Can you work these out from the model? Positions are in its coordinate system, mm. A direction names the side the tool comes from. Round coordinates to 2 decimals unless told otherwise and drop trailing zeros. Write each loop counter-clockwise with the first axis right and the second up, starting at its lowest first coordinate (ties: lowest second). Pieces come first, ordered by that corner, then holes.
Q1. We'd pull the mould along Y, two halves only. Please class faces 1 (the cylindrical face through (-29.414, 9.625, 35.14)), 2 (the flat face through (19, 99, 105)), 3 (the flat face through (5, 200, 42)), 4 (the flat face through (5, 0, 42)): +Y half, -Y half, draft (parallel to the pull), parting line (faces both ways), or undercut.
Q2. If we section it at C-C (z = 49): Please give me the cut outline in (x, y), plus the area to 3 significant figures.
Q3. If we section it at A-A (x = -26): Give the number of separate pieces and of enclosed holes in the cut face, plus the area to 3 significant figures.
Q4. If we section it at B-B (y = 53): Please give me the cut outline in (x, z), plus the area to 4 significant figures.
Q5. For faces 5 (the flat face through (-4, 99, 0)), 6 (the flat face through (0, 99, 75)), 7 (the cylindrical face through (-29.414, 59.625, 35.14)), which set-ups out of +Z, -Z, +X, -X, +Y, -Y let a thin tool reach every point of the face, with its end or its side?
Q6. I'm going to push flat-ended pins straight in: pin 1 Ø9.5 at (x, y) = (24, 75) entering from +Z; pin 2 Ø25 at (x, y) = (-24.5, 126) entering from +Z; pin 3 Ø23 at (x, y) = (-18.5, 140) entering from +Z. Where does each tip first touch, or does it pass through?
Q7. Please list where these lines run through material, in increasing order: line 1 along Y through (x, z) = (24, 94.25); line 2 along Y through (x, z) = (-26, 6.5); line 3 along X through (y, z) = (126, 36).
from build123d import *

# Parameters (mm, degrees)
F0_W           = 39
F0_H           = 60
F1_DEPTH       = 200
F4_D           = 15.5
F4_DEPTH       = 18
F4_TIP         = 4.6566697975
F5_D           = 22
F5_CBORE_D     = 31.5
F5_CBORE_DEPTH = 20


# Not quite as in the source:
# - a feature names something its author has since deleted; it is built from what else it names


with BuildPart() as f1:
    # F0 (on Front) → F1 (new body)
    with BuildSketch(Plane.XZ):
        with Locations((19.5, 75)):
            Rectangle(F0_W, F0_H)
        Polygon((0, 45), (-46, 45), (-46, 0), (39, 0), (39, 45), align=None)
    extrude(amount=-F1_DEPTH)

    # F4
    with Locations(Plane.XY.offset(105)):
        with Locations((24, 25), (24, 75), (24, 125), (24, 175)):
            Hole(F4_D / 2, depth=F4_DEPTH)
            with Locations((0, 0, -(F4_DEPTH + F4_TIP / 2))):  # 118° drill point
                Cone(0, F4_D / 2, F4_TIP, mode=Mode.SUBTRACT)

    # F5 (through all)
    with Locations(Plane.XY.offset(45)):
        with Locations((-26, 25), (-26, 75), (-26, 125), (-26, 175)):
            CounterBoreHole(F5_D / 2, F5_CBORE_D / 2, F5_CBORE_DEPTH)


solid = f1.part
A:
1. face 1: undercut
1. face 2: draft
1. face 3: +Y half
1. face 4: -Y half
2. outline: (0, 0) - (39, 0) - (39, 200) - (0, 200) - close
2. area: 7,800 mm2
3. separate pieces: 5
3. enclosed holes: 0
3. area: 4,280 mm2
4. outline: (-46, 0) - (39, 0) - (39, 105) - (0, 105) - (0, 45) - (-46, 45) - close
4. area: 6,165 mm2
5. face 5: -Z, +X, -X, +Y, -Y
5. face 6: +Z, -X, +Y, -Y
5. face 7: +Z
6. pin 1: stops at z = 85.2
6. pin 2: stops at z = 25
6. pin 3: stops at z = 45
7. line 1: y = 0 to 17.25, 32.75 to 67.25, 82.75 to 117.25, 132.75 to 167.25, 182.75 to 200
7. line 2: y = 0 to 14, 36 to 64, 86 to 114, 136 to 164, 186 to 200
7. line 3: x = -46 to -41.72, -10.28 to 39
